Could you check a few things on this model? Use its own coordinates, in mm. A direction names the side the tool comes from. Give positions to 0.01 mm unless a question says otherwise; leave off trailing zeros. Loops run counter-clockwise (first coordinate to the right, second up) from the corner with the lowest first, then second, coordinate; pieces in that order, holes last. Notation, with made-up numbers: M -6.75,8 L 48.25,8 A27 cw 48.25,46 Z; hole C 64.25,43.5 d8. An arc over 180 degrees is marked long. Answer in a Markdown table with one row per item. Add a question column.
1. I'm going to push flat-ended pins straight in: pin 1 Ø6 at (y, z) = (-32.5, 22) entering from +X; pin 2 Ø3 at (x, z) = (-9, 25) entering from +Y; pin 3 Ø2 at (x, y) = (-18, 28) entering from +Z. Where does each tip first touch, or does it pass through?
2. Thinking about a two-plate mould opening in X: for faces 1 (the cylindrical face through (51.46, 26.76, 22.26)), 2 (the cylindrical face through (-3.755, 11.923, 22.815)), 3 (the cylindrical face through (-0.521, 42.136, 22.675)), 4 (the flat face through (-43, 26, 5)), which applies, released by +X, released by -X, zero draft, split by the parting line, or undercut?
3. If we section it at D-D on z = 14: List the corners of the cut face in (x, y) for me.
4. If we section it at A-A on y = 0: List the corners of the cut face in (x, z) for me, then the cut area to 3 significant figures.
5. If we section it at C-C on z = 8: List the corners of the cut face in (x, y) for me.
6. If we section it at B-B on x = 0: Count the separate pieces of the cut face and the enclosed holes in it, then the cut area to 3 significant figures.
7. Which directions (+Z, -Z, +X, -X, +Y, -Y) give clear straight access to the entire face, cutting with the end or side of a thin tool? Please do faces 5 (the flat face through (21, 21, 10)), 6 (the flat face through (21, -21, 35)), 7 (the flat face through (-11.5, 5.9, 45)).
8. I need wall thicknesses on line 1 along Y through (x, z) = (0, 21.25); line 2 along Y through (x, z) = (-32, 13); line 3 along Y through (x, z) = (31.5, 21). Which ranges of each line are inside material? Lowest first, please. Write a range as from..to.
```python
from build123d import *

# Parameters (mm, degrees)
SKETCH3_R          = 4
CUT_EXTRUDE2_DEPTH = 50


with BuildPart() as part:
    # Sketch1 → Revolve2 (revolve)
    with BuildSketch(Plane(origin=(0, 0, 0), x_dir=(0, 0, -1), z_dir=(1, 0, 0))):
        Polygon((-45, 12.5), (-45, 25), (-35, 27.679491924), (-35, 48.660254038), (-40, 50), (-40, 58), (-5, 58), (-5, 50), (-10, 48.660254038), (-10, 27.679491924), (0, 25), (0, 12.5), align=None)
    revolve(axis=Axis((0, 0, 0), (0, 0, 1)))

    # Sketch3 → Cut-Extrude2 (cut)
    with BuildSketch(Plane.XY.offset(35)):
        with Locations((-33.056079661, -19.084936491)):
            Circle(SKETCH3_R)
        with Locations((0, 38.169872981)):
            Circle(SKETCH3_R)
        with Locations((-33.056079661, 19.084936491)):
            Circle(SKETCH3_R)
        with Locations((0, -38.169872981)):
            Circle(SKETCH3_R)
        with Locations((33.056079661, -19.084936491)):
            Circle(SKETCH3_R)
        with Locations((33.056079661, 19.084936491)):
            Circle(SKETCH3_R)
    extrude(amount=-CUT_EXTRUDE2_DEPTH, mode=Mode.SUBTRACT)


solid = part.part
```
Results:
| question | item | result |
|---|---|---|
| 1 | pin 1 | x = 49.94 |
| 1 | pin 2 | y = 57.51 |
| 1 | pin 3 | z = 35 |
| 2 | face 1 | split by the parting line |
| 2 | face 2 | undercut |
| 2 | face 3 | undercut |
| 2 | face 4 | zero draft |
| 3 | outline | C 0,0 d116; hole C -33.06,-19.08 d8; hole C -33.06,19.08 d8; hole C 0,0 d25; hole C 0,-38.17 d8; hole C 0,38.17 d8; hole C 33.06,-19.08 d8; hole C 33.06,19.08 d8 |
| 4 | outline | M -58,5 L -50,5 L -48.66,10 L -27.68,10 L -25,0 L -12.5,0 L -12.5,45 L -25,45 L -27.68,35 L -48.66,35 L -50,40 L -58,40 Z; M 12.5,0 L 25,0 L 27.68,10 L 48.66,10 L 50,5 L 58,5 L 58,40 L 50,40 L 48.66,35 L 27.68,35 L 25,45 L 12.5,45 Z |
| 4 | area | 3,000 mm2 |
| 5 | outline | C 0,0 d116; C 0,0 d54.29; hole C 0,0 d98.39; hole C 0,0 d25 |
| 6 | separate pieces | 4 |
| 6 | enclosed holes | 0 |
| 6 | area | 2,600 mm2 |
| 7 | face 5 | -Z |
| 7 | face 6 | +Z |
| 7 | face 7 | +Z, +X, -X, +Y, -Y |
| 8 | line 1 | -58..-42.17, -34.17..-12.5, 12.5..34.17, 42.17..58 |
| 8 | line 2 | -48.37..-22.94, -15.23..15.23, 22.94..48.37 |
| 8 | line 3 | -48.7..-22.77, -15.4..15.4, 22.77..48.7 |
